Job drawing, mm, ordinate dimensions from the low corner. One solid piece. A direction names the side the tool comes from. Give positions to 0.01 mm unless a question says otherwise; leave off trailing zeros. Order: outer loops, then holes, each group sorted by start corner. A loop starts at its lowest first (then second) coordinate and runs counter-clockwise, first axis right, second up. Notation, with made-up numbers: M -3.5,0.25 L 22.5,0.25 A26 cw 22.5,22.25 Z; hole C 70.25,74.5 d10. An arc over 180 degrees is marked long. One line per item, written item: value. Start each with the question number.
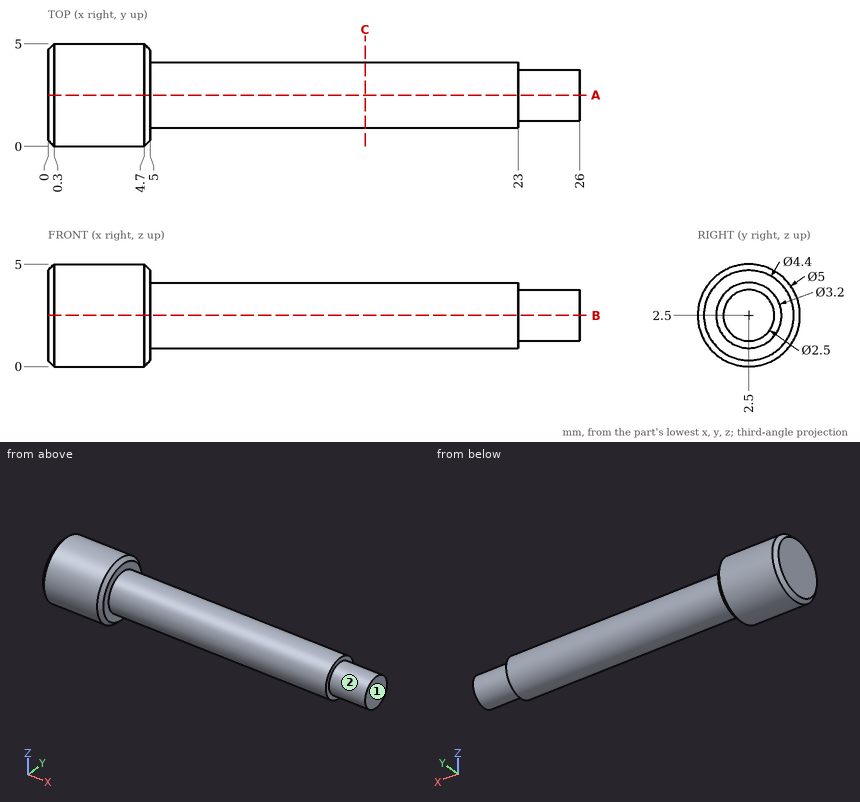
1) Drop flat-ended pins along their axis: P1, Ø3, axis at x = 10.5, z = 4, coming from the +Y side; P2, Ø1.5, axis at x = 6.5, y = 2.5, coming from the +Z side; P3, Ø1.5, axis at x = 23, y = 1, coming from the -Z side. Give the stop position or say it passes through.
2) Slice it at C-C (x = 15.5). List the corners of the cut face in (y, z).
3) Tool access for the marked faces 1 and 2: list every direction of +Z, -Z, +X, -X, +Y, -Y with a clear straight run to the whole face (end or side of a thin tool).
4) Slice it at A-A (y = 2.5). List the corners of the cut face in (x, z), plus the area to 3 significant figures.
5) Drill centre lines: line 1 (Y direction, x = 23.5, z = 2.5); line 2 (X direction, y = 1.05, z = 1); line 3 (X direction, y = 3.8, z = 2.5). Where is each one in solid material? Low to high.
Results list:
1. P1: stops at y = 4.1
1. P2: stops at z = 4.1
1. P3: stops at z = 1.09
2. outline: C 2.5,2.5 d3.2
3. face 1: +Z, -Z, +X, +Y, -Y
3. face 2: +X
4. outline: M 0,0.3 L 0.3,0 L 4.7,0 L 5,0.3 L 5,0.9 L 23,0.9 L 23,1.25 L 26,1.25 L 26,3.75 L 23,3.75 L 23,4.1 L 5,4.1 L 5,4.7 L 4.7,5 L 0.3,5 L 0,4.7 Z
4. area: 89.9 mm²
5. line 1: y = 1.25 to 3.75
5. line 2: x = 0 to 5
5. line 3: x = 0 to 23
